Input: part model. Units: mm. Frame: model coordinates. A direction names the side the tool comes from. Give positions to 0.01 mm unless a question says otherwise; leave off trailing zeros. Loops run counter-clockwise (first coordinate to the right, second up) from the corner with the lowest first, then second, coordinate; pieces in that order, holes last. Notation, with made-up numbers: (65.25, 26) - (113.25, 26) arc R24 ccw to (113.25, 53) - close; hole circle Ø9 at (-1.75, -7). An arc over 180 degrees is marked (long way). One line per item, written item: value.
from build123d import *

# Parameters (mm, degrees)
SKETCH_2_W           = 23.6
SKETCH_2_H           = 16
EXTRUDE_1_DEPTH      = 4
EXTRUDE_START        = 4
EXTRUDE_3_DEPTH      = 4.5
SKETCH_5_R           = 0.3
CUT_EXTRUDE_10_DEPTH = 1
EXTRUDE_2_DEPTH      = 2.5
SKETCH_6_W           = 4
SKETCH_6_H           = 2.95
EXTRUDE_4_DEPTH      = 100
SKETCH_7_R           = 0.7
CUT_EXTRUDE_11_DEPTH = 119.987436312
SKETCH_7_3_R         = 1
SKETCH_7_3_R_2       = 0.7
CUT_EXTRUDE_12_DEPTH = 1
CUT_EXTRUDE_START    = -15
SKETCH_7_4_R         = 1
SKETCH_7_4_R_2       = 0.7
CUT_EXTRUDE_13_DEPTH = 1


with BuildPart() as part:
    # 草图2 → 凸台-拉伸1 (new body)
    with BuildSketch(Plane(origin=(0, 0, 0), x_dir=(0, 0, -1), z_dir=(1, 0, 0))):
        with Locations((5.8, 0)):
            Rectangle(SKETCH_2_W, SKETCH_2_H)
    extrude(amount=EXTRUDE_1_DEPTH)

    # 草图2<10> → 凸台-拉伸3 (add)
    with BuildSketch(Plane(origin=(0, 0, 0), x_dir=(0, 0, -1), z_dir=(1, 0, 0)).offset(EXTRUDE_START)):
        with BuildLine():
            ThreePointArc((0, -1.8), (1.272792206, -1.272792206), (1.8, 0))
            Line((1.8, 0), (0, 0))
            Line((0, 0), (0, -1.8))
        make_face()
        with BuildLine():
            Line((0, 0), (1.8, 0))
            ThreePointArc((1.8, 0), (1.272792206, 1.272792206), (0, 1.8))
            Line((0, 1.8), (0, 0))
        make_face()
        with BuildLine():
            Line((0, -1.8), (0, 0))
            Line((0, 0), (-1.8, 0))
            ThreePointArc((-1.8, 0), (-1.272792206, -1.272792206), (0, -1.8))
        make_face()
        with BuildLine():
            Line((-1.8, 0), (0, 0))
            Line((0, 0), (0, 1.8))
            ThreePointArc((0, 1.8), (-1.272792206, 1.272792206), (-1.8, 0))
        make_face()
    extrude(amount=EXTRUDE_3_DEPTH)

    # 草图5 → 切除-拉伸10 (cut)
    with BuildSketch(Plane(origin=(8.5, 0, 0), x_dir=(0, 0, -1), z_dir=(1, 0, 0))):
        Circle(SKETCH_5_R)
    extrude(amount=-CUT_EXTRUDE_10_DEPTH, mode=Mode.SUBTRACT)

    # 草图2<4> → 凸台-拉伸2 (add)
    with BuildSketch(Plane(origin=(0, 0, 0), x_dir=(0, 0, -1), z_dir=(1, 0, 0)).offset(EXTRUDE_START)):
        with BuildLine():
            ThreePointArc((-3.354101966, 3), (-1.837117307, 4.107919181), (0, 4.5))
            Line((0, 4.5), (-3.968626967, 4.5))
            ThreePointArc((-3.968626967, 4.5), (-4.643360347, 3.799895352), (-5.196152423, 3))
            Line((-5.196152423, 3), (-3.354101966, 3))
        make_face()
        with BuildLine():
            Line((0, 5), (1.8, 5))
            Line((1.8, 5), (1.8, 5.723635209))
            ThreePointArc((1.8, 5.723635209), (-1.245012655, 5.869407422), (-3.968626967, 4.5))
            Line((-3.968626967, 4.5), (0, 4.5))
            Line((0, 4.5), (0, 5))
        make_face()
        with BuildLine():
            ThreePointArc((0, 4.5), (0.919393397, 4.405078408), (1.8, 4.124318125))
            Line((1.8, 4.124318125), (1.8, 5))
            Line((1.8, 5), (0, 5))
            Line((0, 5), (0, 4.5))
        make_face()
        with BuildLine():
            ThreePointArc((1.8, 4.124318125), (3.764970119, 2.464751509), (4.5, 0))
            Line((4.5, 0), (6, 0))
            ThreePointArc((6, 0), (5.286764074, 2.837274331), (3.31662479, 5))
            Line((3.31662479, 5), (1.8, 5))
            Line((1.8, 5), (1.8, 4.124318125))
        make_face()
        with BuildLine():
            Line((1.8, 5.723635209), (1.8, 5))
            Line((1.8, 5), (3.31662479, 5))
            ThreePointArc((3.31662479, 5), (2.583771331, 5.415175501), (1.8, 5.723635209))
        make_face()
        with BuildLine():
            Line((6, 0), (4.5, 0))
            ThreePointArc((4.5, 0), (4.489038226, -0.313904132), (4.456206309, -0.626278954))
            Line((4.456206309, -0.626278954), (3.903880188, -4.556283516))
            ThreePointArc((3.903880188, -4.556283516), (5.262635021, -2.881782892), (5.941608412, -0.835038606))
            ThreePointArc((5.941608412, -0.835038606), (5.985384302, -0.418538842), (6, 0))
        make_face()
        with BuildLine():
            Line((5.356261262, -5), (5.941608412, -0.835038606))
            ThreePointArc((5.941608412, -0.835038606), (5.262635021, -2.881782892), (3.903880188, -4.556283516))
            Line((3.903880188, -4.556283516), (3.841519903, -5))
            Line((3.841519903, -5), (5.356261262, -5))
        make_face()
        Polygon((4.934638757, -8), (5.356261262, -5), (3.841519903, -5), (3.419897399, -8), align=None)
        with BuildLine():
            ThreePointArc((-5.196152423, 3), (-4.643360347, 3.799895352), (-3.968626967, 4.5))
            Line((-3.968626967, 4.5), (-6, 4.5))
            Line((-6, 4.5), (-6, 3))
            Line((-6, 3), (-5.196152423, 3))
        make_face()
    extrude(amount=EXTRUDE_2_DEPTH)

    # 草图6 → 凸台-拉伸4 (add)
    with BuildSketch(Plane(origin=(0, 0, -17.6), x_dir=(-1, 0, 0), z_dir=(0, 0, -1))):
        with Locations((-2, 6.525)):
            Rectangle(SKETCH_6_W, SKETCH_6_H)
        with Locations((-2, -6.525)):
            Rectangle(SKETCH_6_W, SKETCH_6_H)
    extrude(amount=EXTRUDE_4_DEPTH)

    # 镜向1: part across plane


with BuildPart() as part_1:
    add(part.part)
    add(part.part.mirror(Plane(origin=(0, 0, 0), x_dir=(0, 0, 1), z_dir=(1, 0, 0))))

    # 草图7 → 切除-拉伸11 (cut, through all)
    with BuildSketch(Plane(origin=(0, 8, 0), x_dir=(1, 0, 0), z_dir=(0, 1, 0))):
        with Locations(Location((0, 113.6, 0), (0, 0, 270))):
            Circle(SKETCH_7_R)
        with Locations(Location((0, 93.6, 0), (0, 0, 270))):
            Circle(SKETCH_7_R)
    extrude(amount=-CUT_EXTRUDE_11_DEPTH, mode=Mode.SUBTRACT)

    # 草图7<3> → 切除-拉伸12 (cut)
    # profile 1 of 2: a face of its own
    with BuildSketch(Plane(origin=(0, 8, 0), x_dir=(1, 0, 0), z_dir=(0, 1, 0))):
        with Locations(Location((0, 93.6, 0), (0, 0, 270))):
            Circle(SKETCH_7_3_R)
        with Locations(Location((0, 93.6, 0), (0, 0, 270))):
            Circle(SKETCH_7_3_R_2, mode=Mode.SUBTRACT)
    # profile 2 of 2: a face of its own
    with BuildSketch(Plane(origin=(0, 8, 0), x_dir=(1, 0, 0), z_dir=(0, 1, 0))):
        with Locations(Location((0, 113.6, 0), (0, 0, 270))):
            Circle(SKETCH_7_3_R)
        with Locations(Location((0, 113.6, 0), (0, 0, 270))):
            Circle(SKETCH_7_3_R_2, mode=Mode.SUBTRACT)
    extrude(amount=-CUT_EXTRUDE_12_DEPTH, mode=Mode.SUBTRACT)

    # 草图7<4> → 切除-拉伸13 (cut)
    # profile 1 of 2: a face of its own
    with BuildSketch(Plane(origin=(0, 8, 0), x_dir=(1, 0, 0), z_dir=(0, 1, 0)).offset(CUT_EXTRUDE_START)):
        with Locations(Location((0, 93.6, 0), (0, 0, 270))):
            Circle(SKETCH_7_4_R)
        with Locations(Location((0, 93.6, 0), (0, 0, 270))):
            Circle(SKETCH_7_4_R_2, mode=Mode.SUBTRACT)
    # profile 2 of 2: a face of its own
    with BuildSketch(Plane(origin=(0, 8, 0), x_dir=(1, 0, 0), z_dir=(0, 1, 0)).offset(CUT_EXTRUDE_START)):
        with Locations(Location((0, 113.6, 0), (0, 0, 270))):
            Circle(SKETCH_7_4_R)
        with Locations(Location((0, 113.6, 0), (0, 0, 270))):
            Circle(SKETCH_7_4_R_2, mode=Mode.SUBTRACT)
    extrude(amount=-CUT_EXTRUDE_13_DEPTH, mode=Mode.SUBTRACT)


solid = part_1.part
Item 1: Section A-A, the plane x = 2.5. Output: boundary loops of the cut face in (y, z), and give its area (3 significant figures).
Verdict:
outline: (-8, -117.6) - (-5.05, -117.6) - (-5.05, -17.6) - (5.05, -17.6) - (5.05, -117.6) - (8, -117.6) - (8, 6) - (-8, 6) - close
area: 968 mm^2
Item 2: Section B-B, the plane z = -56. Output: boundary loops of the cut face in (x, y), and give its area (3 significant figures).
Verdict:
outline: (-4, -8) - (4, -8) - (4, -5.05) - (-4, -5.05) - close; (-4, 5.05) - (4, 5.05) - (4, 8) - (-4, 8) - close
area: 47.2 mm^2
Item 3: Access query for faces 4 (the face through (0, 5.05, -67)), 5 (the face through (4, -2, 1)), 6 (the face through (-5, 4.5, 5)), 7 (the face through (0, -7.5, -114.6)). Directions: +Z, -Z, +X, -X, +Y, -Y. A direction counts if a zero-diameter tool reaches every point of the face in a straight line with its end or side. Return the directions, or none.
Verdict:
face 4: -Z, +X, -X
face 5: +X
face 6: +Z, -X, +Y
face 7: -Y
Item 4: Section C-C, the plane z = -9.5. Output: boundary loops of the cut face in (x, y), and give its area (3 significant figures).
Verdict:
outline: (-4, -8) - (4, -8) - (4, 8) - (-4, 8) - close
area: 128 mm^2
Item 5: Material intervals for L1, parallel to Y at x = 3.5, z = -30.5; L2, parallel to X at y = 6.65, z = -93.6; L3, parallel to X at y = -3, z = -4.5, sorted ascending.
Verdict:
L1: y = -8 to -5.05, 5.05 to 8
L2: x = -4 to -0.7, 0.7 to 4
L3: x = -6.5 to 6.5
Item 6: Pin query (flat end, axial travel): P1, Ø1.3, axis at x = 0, z = -113.6, coming from the -Y side; P2, Ø8, axis at y = -5.5, z = -82.5, coming from the -X side; P3, Ø1, axis at x = -5.5, z = 5, coming from the +Y side; P4, Ø4, axis at x = -1.5, y = -2, coming from the -Z side. Return the tip coordinate at first contact, or that it passes through.
Verdict:
P1: passes through
P2: stops at x = -4
P3: stops at y = 4.5
P4: stops at z = -17.6
Item 7: Draft query along Y for faces 1 (the face through (-4, -2, 1)), 2 (the face through (-5, 3, 5)), 3 (the face through (0, 7.5, -114.6)). Return one class per face: pulls with the +Y half, pulls with the -Y half, needs draft (parallel to the pull), parting line crosses it, or undercut.
Verdict:
face 1: undercut
face 2: pulls with the -Y half
face 3: needs draft
